Design review of the part built by this model. Coordinates are the model's own, in mm. Face numbers are marked on the shaded views. A direction names the side the tool comes from. Coordinates: 2 decimals unless noted, no trailing zeros. Loops run counter-clockwise (first coordinate to the right, second up) from the corner with the lowest first, then second, coordinate; pieces in that order, holes last. Notation, with made-up numbers: (89, -17.5) -> (112, -17.5) arc R34 cw to (112, 20.5) -> close; hole circle Ø9 at (-6, 0.5). An arc over 180 degrees is marked (long way). Use one line per item in the form item = value. Start each with the question number.
1. For pin 1 (6 mm diameter, centred on x = 32, z = -9, fed in from -Y); pin 2 (2.5 mm diameter, centred on x = 41.656, z = 0, fed in from -Y) (3 decimals); pin 3 (8 mm diameter, centred on y = -13, z = -0.5, fed in from -X); pin 4 (4 mm diameter, centred on x = 30, y = -9.5, fed in from -Z), all flat-tipped, find the tip position at first contact; note any pin that passes through.
2. The part is to be moulded in two halves that separate along Z. For the marked faces 3, 4, 5 and 6, say which applies: released by +Z, released by -Z, zero draft, split by the parting line, or undercut.
3. Consider section A-A (y = 5.25). State the section outline as (x, z) points, then the cut area to 3 significant figures.
4. Machinability: for the marked faces 1 and 2, which of the approach directions +Z, -Z, +X, -X, +Y, -Y give a long, thin tool a straight path to every point of the face, cutting with its end or side? Answer none if there is none.
5. Wall thickness on line 1 (Z direction, x = 0, y = -2.3); line 2 (X direction, y = -11.5, z = 0): over which ranges is each line inside the solid? List them lowest first. Write a range as from..to.
from build123d import *

# Parameters (mm, degrees)
SCREW_HOLES_COUNT = 12


with BuildPart() as part:
    # Cross Section → Main (revolve)
    with BuildSketch(Plane.XY):
        Polygon((-38.1, 0), (-38.1, -3.175), (-39.6875, -3.175), (-39.6875, -15.875), (-40.0685, -15.215088642), (-40.0685, -3.175), (-46.9265, -3.175), (-46.9265, 9.525), (-45.339, 9.525), (-45.339, 0), align=None)
    revolve(axis=Axis((0, 55, 0), (0, -1, 0)))

    # Sketch7 → #3-48 Tapped Hole1 (revolve, cut)
    with BuildSketch(Plane(origin=(-41.656, 0, 0), x_dir=(0, 0, 1), z_dir=(1, 0, 0))):
        Polygon((0, 0), (0, 3.901027994), (0.99695, 3.302), (0.99695, 0), align=None)
    f_3_48_tapped_hole1 = revolve(axis=Axis((-41.656, 6.35, 0), (0, -1, 0)), mode=Mode.SUBTRACT)

    # Screw Holes: #3-48 Tapped Hole1 ×12 about axis
    screw_holes_axis = Axis((0, 0, 0), (0, 1, 0))
    for i in range(1, SCREW_HOLES_COUNT):
        add(f_3_48_tapped_hole1.rotate(screw_holes_axis, i * 360 / SCREW_HOLES_COUNT), mode=Mode.SUBTRACT)


solid = part.part
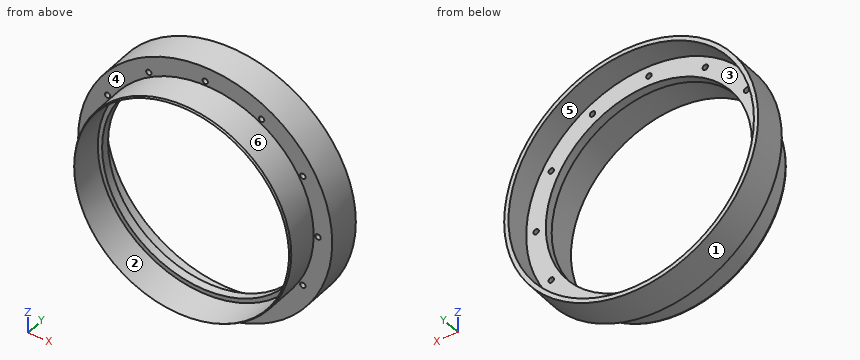
Geometry check:
q1.pin_1 = through
q1.pin_2 = -3.175
q1.pin_3 = -40.07
q1.pin_4 = -28.66
q2.face_3 = undercut
q2.face_4 = zero draft
q2.face_5 = undercut
q2.face_6 = split by the parting line
q3.outline = circle Ø93.85 at (0, 0); hole circle Ø90.68 at (0, 0)
q3.area = 460 mm²
q4.face_1 = +Y, -Y
q4.face_2 = -Y
q5.line_1 = -46.93..-42.65, -40.66..-38.1, 38.1..40.66, 42.65..46.93
q5.line_2 = -40.07..-39.69, 39.69..40.07
